Can you work these out from the model? Positions are in its coordinate system, mm. Face numbers are marked on the shaded views. A direction names the side the tool comes from. Round coordinates to 2 decimals unless told otherwise and drop trailing zeros. Order: outer loops, then holes, each group sorted by start corner. A loop starts at its lowest first (then second) coordinate and runs counter-clockwise, first axis right, second up. Notation, with made-up numbers: (75, 61.5) -> (102, 61.5) arc R19 ccw to (102, 70.5) -> close; hole circle Ø1 at (80.25, 65.5). An arc over 180 degrees is marked (long way). One line per item, written item: value.
```python
from build123d import *

# Parameters (mm, degrees)
SKETCH1_W           = 119.38
SKETCH1_H           = 25.4
BOSS_EXTRUDE1_DEPTH = 12.7
BOSS_EXTRUDE2_DEPTH = 12.7
LPATTERN1_COUNT     = 12
LPATTERN1_PITCH     = 9.4742


with BuildPart() as part:
    # Sketch1 → Boss-Extrude1 (new body)
    with BuildSketch(Plane(origin=(0, 0, 0), x_dir=(1, 0, 0), z_dir=(0, 1, 0))):
        Rectangle(SKETCH1_W, SKETCH1_H)
    extrude(amount=BOSS_EXTRUDE1_DEPTH)

    # Sketch1_4 → Boss-Extrude2 (add)
    with BuildSketch(Plane(origin=(0, 0, 0), x_dir=(1, 0, 0), z_dir=(0, 1, 0))):
        with BuildLine():
            Line((51.816, 13.908285481), (51.816, 12.7))
            Line((51.816, 12.7), (56.388, 12.7))
            Line((56.388, 12.7), (56.388, 13.908285481))
            ThreePointArc((56.388, 13.908285481), (55.997429107, 16.372543207), (54.864, 18.595255564))
            Line((54.864, 18.595255564), (53.34, 18.595255564))
            ThreePointArc((53.34, 18.595255564), (52.206570893, 16.372543207), (51.816, 13.908285481))
        make_face()
    boss_extrude2 = extrude(amount=BOSS_EXTRUDE2_DEPTH)

    # LPattern1: Boss-Extrude2 ×12
    with Locations(*[(-i * LPATTERN1_PITCH, 0, 0) for i in range(1, LPATTERN1_COUNT)]):
        add(boss_extrude2)


solid = part.part
```
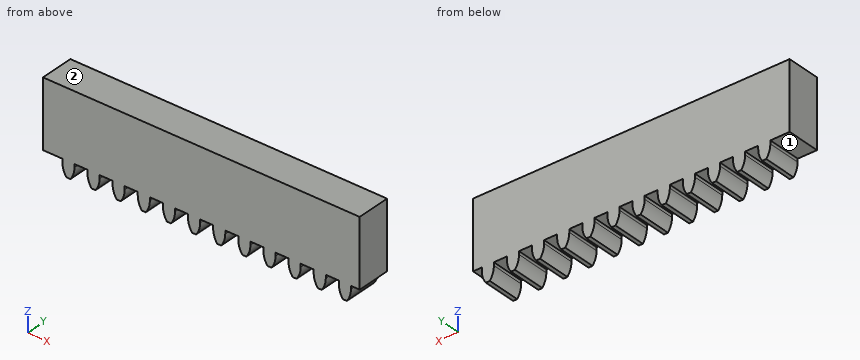
Q1. I want a section at A-A on x = 1.5. List the corners of the cut face in (y, z) for me.
Answers below:
outline: (0, -12.7) -> (12.7, -12.7) -> (12.7, 12.7) -> (0, 12.7) -> close
Q2. On a 3-axis mill with a long thin cutter (end or side, diameter ignored), from which of +Z, -Z, +X, -X, +Y, -Y can I reach the whole of each face in a straight line? I mean the marked faces 1 and 2. Say none if no direction works.
Answers below:
face 1: -Z, -X, +Y, -Y
face 2: +Z, +X, -X, +Y, -Y
Q3. Will these pins go through, and if not, where does the flat tip stop? pin 1 Ø1.3 at (y, z) = (9, -13.5) entering from +X; pin 2 Ø1.3 at (y, z) = (3.5, -13.5) entering from -X; pin 3 Ø5 at (x, y) = (-8.5, 10.5) entering from -Z.
Answers below:
pin 1: x = 56.39
pin 2: x = -52.4
pin 3: z = -17.89
Q4. Please list where these lines run through material, in increasing order: line 1 along Z through (x, y) = (-6.5, 6.5); line 2 along Z through (x, y) = (43, 3).
Answers below:
line 1: -12.7 to 12.7
line 2: -17.08 to 12.7
